```python
from build123d import *

# Parameters (mm, degrees)
BOSS_EXTRUDE1_DEPTH     = 50.8
CUT_EXTRUDE1_DEPTH      = 63.223284049
CUT_EXTRUDE1_DEPTH_BACK = 63.223284049
SKETCH2_R               = 3.175
FILLET1_R               = 3.81


with BuildPart() as part:
    # Sketch1 → Boss-Extrude1 (new body)
    with BuildSketch(Plane(origin=(0, 0, 0), x_dir=(0, 0, -1), z_dir=(1, 0, 0))):
        with BuildLine():
            Line((9.525, 16.130124961), (9.525, 29.677791118))
            Line((9.525, 29.677791118), (11.049, 29.677791118))
            Line((11.049, 29.677791118), (11.049, 16.977791118))
            ThreePointArc((11.049, 16.977791118), (0, -20.2565), (-11.049, 16.977791118))
            Line((-11.049, 16.977791118), (-11.049, 29.677791118))
            Line((-11.049, 29.677791118), (-9.525, 29.677791118))
            Line((-9.525, 29.677791118), (-9.525, 16.130124961))
            ThreePointArc((-9.525, 16.130124961), (0, -18.7325), (9.525, 16.130124961))
        make_face()
    extrude(amount=BOSS_EXTRUDE1_DEPTH)

    # Sketch2 → Cut-Extrude1 (cut, two sides: drawn at the far end of the back side and taken through both)
    with BuildSketch(Plane.XY.offset(-CUT_EXTRUDE1_DEPTH_BACK)):
        with Locations(Location((6.35, 23.327791118, 0), (0, 0, 270))):
            Circle(SKETCH2_R)
        with Locations(Location((44.45, 23.327791118, 0), (0, 0, 270))):
            Circle(SKETCH2_R)
    extrude(amount=CUT_EXTRUDE1_DEPTH + CUT_EXTRUDE1_DEPTH_BACK, mode=Mode.SUBTRACT)

    # Fillet1
    fillet1_edges = [part.edges().sort_by_distance(p)[0] for p in [
        (0, 29.677791118, 10.287),
        (50.8, 29.677791118, 10.287),
        (25.4, 16.130124961, -9.525),
        (25.4, 16.977791118, -11.049),
        (25.4, 16.977791118, 11.049),
        (25.4, 16.130124961, 9.525),
        (50.8, 29.677791118, -10.287),
        (0, 29.677791118, -10.287),
    ]]
    fillet(fillet1_edges, radius=FILLET1_R)


solid = part.part
```
Part model, mm, in its own coordinate system. A direction names the side the tool comes from. Round coordinates to 2 decimals unless told otherwise and drop trailing zeros. Loops run counter-clockwise (first coordinate to the right, second up) from the corner with the lowest first, then second, coordinate; pieces in that order, holes last. Notation, with made-up numbers: (-13.5, 20) -> (28.5, 20) arc R22 cw to (28.5, 52) -> close; hole circle Ø10 at (-37, 26). An arc over 180 degrees is marked (long way). Use a Markdown table: item, result.
1) Cut at D-D, the plane y = 21.5. List the corners of the cut face in (x, z) (3 decimals), and give its area (3 significant figures).
The answers:
| item | result |
|---|---|
| outline | (0, -11.049) -> (3.754, -11.049) -> (3.754, -9.525) -> (0, -9.525) -> close; (0, 9.525) -> (3.754, 9.525) -> (3.754, 11.049) -> (0, 11.049) -> close; (8.946, -11.049) -> (41.854, -11.049) -> (41.854, -9.525) -> (8.946, -9.525) -> close; (8.946, 9.525) -> (41.854, 9.525) -> (41.854, 11.049) -> (8.946, 11.049) -> close; (47.046, -11.049) -> (50.8, -11.049) -> (50.8, -9.525) -> (47.046, -9.525) -> close; (47.046, 9.525) -> (50.8, 9.525) -> (50.8, 11.049) -> (47.046, 11.049) -> close |
| area | 123 mm2 |
2) Pull direction X, two halves, no side cores. Call faces 5 (the cylindrical face through (25.756, 17.244, 11.443)), 6 (the cylindrical face through (1.086, 28.532, 10.276)), 7 (the cylindrical face through (6.5, 26.5, 10.3)), 8 (the flat face through (50.8, -6, 18)): pulls with the +X half, pulls with the -X half, needs draft (parallel to the pull), parting line crosses it, or undercut.
The answers:
| item | result |
|---|---|
| face 5 | needs draft |
| face 6 | pulls with the -X half |
| face 7 | undercut |
| face 8 | pulls with the +X half |
3) Tool access for faces 1 (the flat face through (25, 24, 9.525)), 2 (the flat face through (25, 24, -11.049)), 3 (the cylindrical face through (25.756, 16.476, -9.925)), 4 (the flat face through (25, 29.678, 10)): list every direction of +Z, -Z, +X, -X, +Y, -Y with a clear straight run to the whole face (end or side of a thin tool).
The answers:
| item | result |
|---|---|
| face 1 | +X, -X, +Y |
| face 2 | -Z, +X, -X, +Y |
| face 3 | +X, -X |
| face 4 | +Z, -Z, +X, -X, +Y |
4) Drop flat-ended pins along their axis: pin 1 Ø6 at (x, z) = (44.5, 0.5) entering from +Y; pin 2 Ø1 at (x, y) = (17, -14.5) entering from +Z; pin 3 Ø3.5 at (x, y) = (13, 25) entering from -Z. Give the stop position or say it passes through.
The answers:
| item | result |
|---|---|
| pin 1 | stops at y = -18.4 |
| pin 2 | stops at z = 14.64 |
| pin 3 | stops at z = -11.05 |
5) Probe line 1 (Z direction, x = 40, y = 0); line 2 (Z direction, x = 15, y = 21) (3 decimals); line 3 (Y direction, x = 44, z = 10). List the from-to ranges inside material, lowest first. Write a range as [from, to].
The answers:
| item | result |
|---|---|
| line 1 | z = [-20.26, -18.73], [18.73, 20.26] |
| line 2 | z = [-11.049, -9.525], [9.525, 11.049] |
| line 3 | y = [-17.62, -15.84], [16.33, 20.18], [26.47, 29.68] |
6) Cut at B-B, the plane y = 0. List the corners of the cut face in (x, z).
The answers:
| item | result |
|---|---|
| outline | (0, -20.26) -> (50.8, -20.26) -> (50.8, -18.73) -> (0, -18.73) -> close; (0, 18.73) -> (50.8, 18.73) -> (50.8, 20.26) -> (0, 20.26) -> close |
7) Cut at C-C, the plane z = -17. List the corners of the cut face in (x, y).
The answers:
| item | result |
|---|---|
| outline | (0, -11.01) -> (50.8, -11.01) -> (50.8, -7.87) -> (0, -7.87) -> close; (0, 7.87) -> (50.8, 7.87) -> (50.8, 11.01) -> (0, 11.01) -> close |
8) Cut at A-A, the plane x = 6.35. List the corners of the cut face in (y, z) (1 decimal), and give its area (3 significant figures).
The answers:
| item | result |
|---|---|
| outline | (15.1, -11.1) arc R18.7 cw (long way) to (15.1, 11.1) arc R3.8 ccw to (18.2, 9.5) -> (20.2, 9.5) -> (20.2, 11) -> (18.9, 11) arc R3.8 cw to (15.9, 12.5) arc R20.3 ccw (long way) to (15.9, -12.5) arc R3.8 cw to (18.9, -11) -> (20.2, -11) -> (20.2, -9.5) -> (18.2, -9.5) arc R3.8 ccw to start; (26.5, -11) -> (29.7, -11) -> (29.7, -9.5) -> (26.5, -9.5) -> close; (26.5, 9.5) -> (29.7, 9.5) -> (29.7, 11) -> (26.5, 11) -> close |
| area | 174 mm2 |
